Check sheet for the drawn part. Datum: minimum x, y, z corner. Units: mm. Coordinates: 2 decimals unless noted, no trailing zeros. Write each loop counter-clockwise with the first axis right and the second up, starting at its lowest first coordinate (ties: lowest second). Pieces come first, ordered by that corner, then holes. Notation, with made-up numbers: (-16, 39.25) -> (-2, 39.25) arc R28 ccw to (-2, 73.25) -> close; hole circle Ø2 at (52, -10.75). An arc over 180 degrees is marked (long way). Write item = value, one per line. Start each with the question number.
(1) Section check C-C (z = 28). State how many separate pieces and enclosed holes the cut face has, plus the area to 3 significant figures.
(2) Gauge pin test, flat ends, axial feed: pin 1 Ø8 at (y, z) = (14.5, 29.5) entering from -X (1 decimal); pin 2 Ø4 at (x, z) = (10.5, 17.5) entering from +Y; pin 3 Ø3 at (x, z) = (46, 24) entering from -Y. Record the tip position at first contact, or that the pin passes through.
(3) Material ranges on probe 1 along X at (y, z) = (33, 31.5) (1 decimal); probe 2 along Y at (x, z) = (50.8, 16); probe 3 along Y at (x, z) = (70, 8) (1 decimal), recorded low to high. Write a range as [from, to].
(4) Mould release check, pull along X, two halves, no side actions. Record for the marked faces 1, 2 and 3: released by +X, released by -X, zero draft, split by the parting line, or undercut.
(5) Section check A-A (x = 50.8). Record the cut outline in (y, z), plus the area to 4 significant figures.
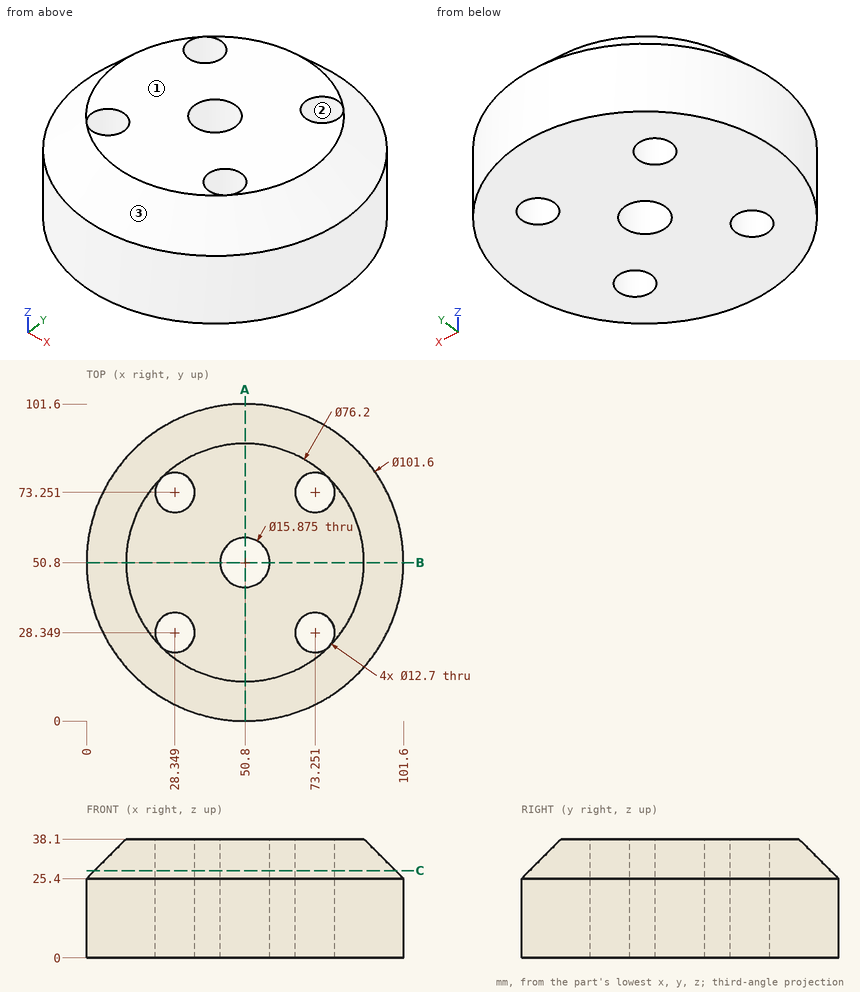
Response:
q1.separate_pieces = 1
q1.enclosed_holes = 5
q1.area = 6,590 mm2
q2.pin_1 = 14.2
q2.pin_2 = 84.17
q2.pin_3 = 0.11
q3.probe_1 = [9.8, 24], [32.7, 68.9], [77.6, 91.8]
q3.probe_2 = [0, 42.86], [58.74, 101.6]
q3.probe_3 = [3.8, 22.9], [33.8, 67.8], [78.7, 97.8]
q4.face_1 = zero draft
q4.face_2 = undercut
q4.face_3 = split by the parting line
q5.outline = (0, 0) -> (42.86, 0) -> (42.86, 38.1) -> (12.7, 38.1) -> (0, 25.4) -> close; (58.74, 0) -> (101.6, 0) -> (101.6, 25.4) -> (88.9, 38.1) -> (58.74, 38.1) -> close
q5.area = 3,105 mm2
